Read the model definition and answer for the solid it produces. Units are mm, in the model's axes. Face numbers are marked on the shaded views. A direction names the side the tool comes from. Coordinates: 2 decimals unless noted, no trailing zeros. Write each loop counter-clockwise with the first axis right and the second up, starting at its lowest first coordinate (ties: lowest second). Pieces come first, ordered by that corner, then holes.
(1) Find the intervals of material crossed by probe 1 along Z at (x, y) = (-8, 29); probe 2 along X at (y, z) = (2.5, 80.5); probe 3 along Y at (x, z) = (3, 192), in increasing order.
(2) Section C-C on z = 430 is taken. Write down the section's boundary in (x, y).
(3) Section A-A on x = 0 is taken. Write down the section's boundary in (y, z), then the cut area to 3 significant figures.
(4) Given pin 1 (12 mm diameter, centred on x = 8, y = 36.5, fed in from -Z); pin 2 (1.5 mm diameter, centred on x = -16.5, y = -4.5, fed in from -Z); pin 3 (1.5 mm diameter, centred on y = -23, z = 334, fed in from +X); pin 4 (2 mm diameter, centred on x = -25, y = 18.5, fed in from +Z), each flat-ended and moving along its own axis, determine where each tip first touches the part or whether it passes through.
(5) Which of the six approach directions +Z, -Z, +X, -X, +Y, -Y give full straight-line access (tool end or side, diameter ignored) to the marked faces 1 and 2?
(6) Section D-D on y = -35 is taken. Write down the section's boundary in (x, z), then the cut area to 3 significant figures.
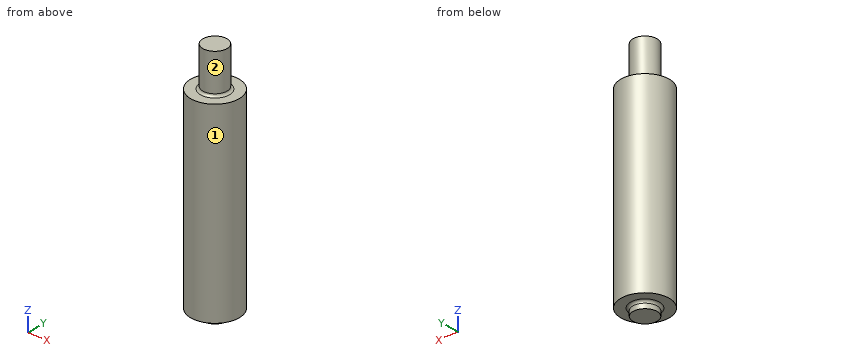
from build123d import *

# Parameters (mm, degrees)
SKETCH1_R           = 25
BOSS_EXTRUDE1_DEPTH = 15
SKETCH2_R           = 50
BOSS_EXTRUDE2_DEPTH = 397
SKETCH3_R           = 25
BOSS_EXTRUDE3_DEPTH = 82
FILLET1_R           = 5


with BuildPart() as part:
    # Sketch1 → Boss-Extrude1 (new body)
    with BuildSketch(Plane.XY):
        Circle(SKETCH1_R)
    extrude(amount=BOSS_EXTRUDE1_DEPTH)

    # Sketch2 → Boss-Extrude2 (add)
    with BuildSketch(Plane.XY.offset(15)):
        Circle(SKETCH2_R)
    extrude(amount=BOSS_EXTRUDE2_DEPTH)

    # Sketch3 → Boss-Extrude3 (add)
    with BuildSketch(Plane.XY.offset(412)):
        Circle(SKETCH3_R)
    extrude(amount=BOSS_EXTRUDE3_DEPTH)

    # Fillet1
    fillet1_edges = [part.edges().sort_by_distance(p)[0] for p in [
        (-25, 0, 15),
        (-25, 0, 412),
    ]]
    fillet(fillet1_edges, radius=FILLET1_R)


solid = part.part
Response:
1. probe 1: z = 15 to 412
1. probe 2: x = -49.94 to 49.94
1. probe 3: y = -49.91 to 49.91
2. outline: circle Ø50 at (0, 0)
3. outline: (-50, 15) - (-30, 15) arc R5 cw to (-25, 10) - (-25, 0) - (25, 0) - (25, 10) arc R5 cw to (30, 15) - (50, 15) - (50, 412) - (30, 412) arc R5 cw to (25, 417) - (25, 494) - (-25, 494) - (-25, 417) arc R5 cw to (-30, 412) - (-50, 412) - close
3. area: 44,600 mm2
4. pin 1: stops at z = 15
4. pin 2: stops at z = 0
4. pin 3: stops at x = 44.78
4. pin 4: stops at z = 412
5. face 1: +Z, -Z
5. face 2: +Z
6. outline: (-35.71, 15) - (35.71, 15) - (35.71, 412) - (-35.71, 412) - close
6. area: 28,400 mm2
